Geometry: final body of the model. Coordinates: model frame, mm. A direction names the side the tool comes from. Give positions to 0.01 mm unless a question says otherwise; leave off trailing zeros. Loops run counter-clockwise (first coordinate to the right, second up) from the corner with the lowest first, then second, coordinate; pieces in that order, holes last.
from build123d import *

# Parameters (mm, degrees)
SKETCH1_W           = 150
SKETCH1_H           = 70
BOSS_EXTRUDE1_DEPTH = 4.5
SKETCH7_W           = 4
SKETCH7_H           = 150
BOSS_EXTRUDE2_DEPTH = 4
SKETCH8_R           = 1.95
CUT_EXTRUDE5_DEPTH  = 10
SKETCH9_R           = 1.65
CUT_EXTRUDE6_DEPTH  = 166.747549001
SKETCH10_R          = 3
CUT_EXTRUDE7_DEPTH  = 1.5
SKETCH13_R          = 2.1
CUT_EXTRUDE10_DEPTH = 0.5
SKETCH14_R          = 1.1
SKETCH14_W          = 3.4
SKETCH14_H          = 9.2
CUT_EXTRUDE11_DEPTH = 166.747549001
FILLET3_R           = 1.5
SKETCH15_W          = 12
SKETCH15_H          = 27
CUT_EXTRUDE12_DEPTH = 2.5
FILLET4_R           = 4


with BuildPart() as part:
    # Sketch1 → Boss-Extrude1 (new body)
    with BuildSketch(Plane(origin=(0, 0, 0), x_dir=(0, 1, 0), z_dir=(0, 0, 1))):
        with Locations((75, 35)):
            Rectangle(SKETCH1_W, SKETCH1_H)
    extrude(amount=BOSS_EXTRUDE1_DEPTH)

    # Sketch7 → Boss-Extrude2 (add)
    with BuildSketch(Plane(origin=(0, 0, 0), x_dir=(1, 0, 0), z_dir=(0, 0, -1))):
        with Locations((-2, -75)):
            Rectangle(SKETCH7_W, SKETCH7_H)
    extrude(amount=BOSS_EXTRUDE2_DEPTH)

    # Sketch8 → Cut-Extrude5 (cut)
    with BuildSketch(Plane.YZ):
        with Locations(Location((15, 0.025, 0), (0, 0, 270))):
            Circle(SKETCH8_R)
        with Locations(Location((75, 0.125, 0), (0, 0, 270))):
            Circle(SKETCH8_R)
        with Locations(Location((135, 0.225, 0), (0, 0, 270))):
            Circle(SKETCH8_R)
    extrude(amount=-CUT_EXTRUDE5_DEPTH, mode=Mode.SUBTRACT)

    # Sketch9 → Cut-Extrude6 (cut, through all)
    with BuildSketch(Plane.XY.offset(4.5)):
        with Locations((-66, 146)):
            Circle(SKETCH9_R)
        with Locations((-66, 4)):
            Circle(SKETCH9_R)
    extrude(amount=-CUT_EXTRUDE6_DEPTH, mode=Mode.SUBTRACT)

    # Sketch10 → Cut-Extrude7 (cut)
    with BuildSketch(Plane.XY.offset(4.5)):
        with Locations((-66, 146)):
            Circle(SKETCH10_R)
        with Locations((-66, 4)):
            Circle(SKETCH10_R)
    extrude(amount=-CUT_EXTRUDE7_DEPTH, mode=Mode.SUBTRACT)

    # Sketch13 → Cut-Extrude10 (cut)
    with BuildSketch(Plane.XY.offset(4.5)):
        with Locations((-20, 28.25)):
            Circle(SKETCH13_R)
        with Locations((-20, 11.75)):
            Circle(SKETCH13_R)
    extrude(amount=-CUT_EXTRUDE10_DEPTH, mode=Mode.SUBTRACT)

    # Sketch14 → Cut-Extrude11 (cut, through all)
    with BuildSketch(Plane.XY.offset(4.5)):
        with Locations((-20, 11.75)):
            Circle(SKETCH14_R)
        with Locations((-20, 28.25)):
            Circle(SKETCH14_R)
        with Locations((-20, 20)):
            Rectangle(SKETCH14_W, SKETCH14_H)
    extrude(amount=-CUT_EXTRUDE11_DEPTH, mode=Mode.SUBTRACT)

    # Fillet3
    fillet3_edges = [part.edges().sort_by_distance(p)[0] for p in [
        (-18.3, 24.6, 2.25),
        (-18.3, 15.4, 2.25),
        (-21.7, 15.4, 2.25),
        (-21.7, 24.6, 2.25),
    ]]
    fillet(fillet3_edges, radius=FILLET3_R)

    # Sketch15 → Cut-Extrude12 (cut)
    with BuildSketch(Plane(origin=(0, 0, 0), x_dir=(1, 0, 0), z_dir=(0, 0, -1))):
        with Locations((-20, -20)):
            Rectangle(SKETCH15_W, SKETCH15_H)
    extrude(amount=-CUT_EXTRUDE12_DEPTH, mode=Mode.SUBTRACT)

    # Fillet4
    fillet4_edges = [part.edges().sort_by_distance(p)[0] for p in [
        (-14, 6.5, 1.25),
        (-14, 33.5, 1.25),
        (-26, 33.5, 1.25),
        (-26, 6.5, 1.25),
    ]]
    fillet(fillet4_edges, radius=FILLET4_R)


solid = part.part
Item 1: Draft query along X for faces 1 (the face through (-17, 20, 2.5)), 2 (the face through (0, 76, 2)), 3 (the face through (-66.4, 144.4, 1.5)), 4 (the face through (-35, 74, 4.5)). Return one class per face: +X half, -X half, draft (parallel to the pull), parting line (faces both ways), or undercut.
Values follow:
face 1: undercut
face 2: +X half
face 3: undercut
face 4: draft
Item 2: Pin query (flat end, axial travel): pin 1 (1.5 mm diameter, centred on y = 62.5, z = -0.5, fed in from -X); pin 2 (1.7 mm diameter, centred on y = 74.5, z = 0.5, fed in from +X); pin 3 (2 mm diameter, centred on x = -10, y = 120.5, fed in from -Z); pin 4 (4.5 mm diameter, centred on x = -66, y = 146, fed in from +Z). Return the tip coordinate at first contact, or that it passes through.
Values follow:
pin 1: stops at x = -70
pin 2: stops at x = -10
pin 3: stops at z = 0
pin 4: stops at z = 3
Item 3: Ray query, probe 1 along Y at (x, z) = (-66, 1.8); probe 2 along Y at (x, z) = (-66, 4.1); probe 3 along Y at (x, z) = (-20, 4.35). Return the intervals inside material, ascending.
Values follow:
probe 1: y = 0 to 2.35, 5.65 to 144.35, 147.65 to 150
probe 2: y = 0 to 1, 7 to 143, 149 to 150
probe 3: y = 0 to 9.65, 13.85 to 15.4, 24.6 to 26.15, 30.35 to 150
Item 4: Section query D-D on x = -7. Return loops of the section in (y, z) (3 decimals), plus the area to 3 significant figures.
Values follow:
outline: (0, 0) - (13.05, 0) arc R1.95 cw (long way) to (16.95, 0) - (73.054, 0) arc R1.95 cw (long way) to (76.946, 0) - (133.063, 0) arc R1.95 cw (long way) to (136.937, 0) - (150, 0) - (150, 4.5) - (0, 4.5) - close
area: 656 mm2
Item 5: Set-up query: faces 5 (the face through (-3.819, 135.086, 2.173)), 6 (the face through (-37, 74, 0)), 7 (the face through (-20, 33.5, 1)), 8 (the face through (-64.7, 2.7, 3)). Return all of +Z, -Z, +X, -X, +Y, -Y with unobstructed straight access to the full face (end or side cutting, diameter ignored); none if empty.
Values follow:
face 5: +X
face 6: -Z, -X, +Y, -Y
face 7: -Z
face 8: +Z
Item 6: Section query B-B on x = -66. Return loops of the section in (y, z).
Values follow:
outline: (0, 0) - (2.35, 0) - (2.35, 3) - (1, 3) - (1, 4.5) - (0, 4.5) - close; (5.65, 0) - (144.35, 0) - (144.35, 3) - (143, 3) - (143, 4.5) - (7, 4.5) - (7, 3) - (5.65, 3) - close; (147.65, 0) - (150, 0) - (150, 4.5) - (149, 4.5) - (149, 3) - (147.65, 3) - close
Item 7: Section query C-C on y = 135. Return loops of the section in (x, z) (3 decimals), plus the area to 3 significant figures.
Values follow:
outline: (-70, 0) - (-10, 0) - (-10, 2.175) - (0, 2.175) - (0, 4.5) - (-70, 4.5) - close; (-4, -4) - (0, -4) - (0, -1.725) - (-4, -1.725) - close
area: 302 mm2
Item 8: Section query A-A on y = 75. Return loops of the section in (x, z) (3 decimals), plus the area to 3 significant figures.
Values follow:
outline: (-70, 0) - (-10, 0) - (-10, 2.075) - (0, 2.075) - (0, 4.5) - (-70, 4.5) - close; (-4, -4) - (0, -4) - (0, -1.825) - (-4, -1.825) - close
area: 303 mm2
